from build123d import *

# Parameters (mm, degrees)
SKETCH1_R                                     = 50.8
BOSS_EXTRUDE1_DEPTH                           = 3.175
BOSS_EXTRUDE2_DEPTH                           = 3.175
FILLET1_R                                     = 3.175
CSK_FOR_8_FLAT_HEAD_SOCKET_CAP_SCREW1_A_COUNT = 2
CSK_FOR_8_FLAT_HEAD_SOCKET_CAP_SCREW1_A_PITCH = 23.8125
CSK_FOR_8_FLAT_HEAD_SOCKET_CAP_SCRE_2_COUNT   = 2
CSK_FOR_8_FLAT_HEAD_SOCKET_CAP_SCRE_2_PITCH   = 65.445830702
CSK_FOR_8_FLAT_HEAD_SOCKET_CAP_SCRE_3_COUNT   = 2
CSK_FOR_8_FLAT_HEAD_SOCKET_CAP_SCRE_3_PITCH   = 60.96
CIRPATTERN1_COUNT                             = 6
CSK_FOR_4_FLAT_HEAD_SOCKET_CAP_SCREW2_A_COUNT = 2
CSK_FOR_4_FLAT_HEAD_SOCKET_CAP_SCREW2_A_PITCH = 15.875
CSK_FOR_4_FLAT_HEAD_SOCKET_CAP_SCRE_2_COUNT   = 2
CSK_FOR_4_FLAT_HEAD_SOCKET_CAP_SCRE_2_PITCH   = 15.875
SKETCH17_W                                    = 12.7
SKETCH17_H                                    = 25.4
CUT_EXTRUDE2_DEPTH                            = 74.042253397
FILLET2_R                                     = 1.5875


with BuildPart() as part:
    # Sketch1 → Boss-Extrude1 (new body)
    with BuildSketch(Plane(origin=(0, 0, 0), x_dir=(1, 0, 0), z_dir=(0, 1, 0))):
        with Locations(Location((0, 0, 0), (0, 0, 270))):
            Circle(SKETCH1_R)
    extrude(amount=BOSS_EXTRUDE1_DEPTH)

    # Sketch8 → Boss-Extrude2 (add)
    with BuildSketch(Plane.XZ):
        with BuildLine():
            Line((-52.3875, -15.875), (-48.255822188, -15.875))
            ThreePointArc((-48.255822188, -15.875), (-50.8, 0), (-48.255822188, 15.875))
            Line((-48.255822188, 15.875), (-52.3875, 15.875))
            Line((-52.3875, 15.875), (-52.3875, -15.875))
        make_face()
    extrude(amount=-BOSS_EXTRUDE2_DEPTH)

    # Fillet1
    fillet1_edges = [part.edges().sort_by_distance(p)[0] for p in [
        (-48.255822188, 1.5875, 15.875),
        (-48.255822188, 1.5875, -15.875),
    ]]
    fillet(fillet1_edges, radius=FILLET1_R)

    # Sketch6 → CSK for #8 Flat Head Socket Cap Screw1 (revolve, cut)
    with BuildSketch(Plane(origin=(-44.45, 0, 11.90625), x_dir=(0, 0, -1), z_dir=(1, 0, 0))):
        Polygon((0, 0), (0, 3.175), (2.2479, 3.175), (2.2479, 2.658961536), (4.5593, 0), align=None)
    csk_for_8_flat_head_socket_cap_screw1 = revolve(axis=Axis((-44.45, -6.35, 11.90625), (0, 1, 0)), mode=Mode.SUBTRACT)

    # CSK for #8 Flat Head Socket Cap Screw1 a: CSK for #8 Flat Head Socket Cap Screw1 ×2
    with Locations(*[(0, 0, -i * CSK_FOR_8_FLAT_HEAD_SOCKET_CAP_SCREW1_A_PITCH) for i in range(1, CSK_FOR_8_FLAT_HEAD_SOCKET_CAP_SCREW1_A_COUNT)]):
        add(csk_for_8_flat_head_socket_cap_screw1, mode=Mode.SUBTRACT)

    # CSK for _8 Flat Head Socket Cap Scre 2: CSK for #8 Flat Head Socket Cap Screw1 ×2
    with Locations(*[Vector(0.9314573494796193, 0, -0.36385052714047633) * (i * CSK_FOR_8_FLAT_HEAD_SOCKET_CAP_SCRE_2_PITCH) for i in range(1, CSK_FOR_8_FLAT_HEAD_SOCKET_CAP_SCRE_2_COUNT)]):
        add(csk_for_8_flat_head_socket_cap_screw1, mode=Mode.SUBTRACT)

    # CSK for _8 Flat Head Socket Cap Scre 3: CSK for #8 Flat Head Socket Cap Screw1 ×2
    with Locations(*[(i * CSK_FOR_8_FLAT_HEAD_SOCKET_CAP_SCRE_3_PITCH, 0, 0) for i in range(1, CSK_FOR_8_FLAT_HEAD_SOCKET_CAP_SCRE_3_COUNT)]):
        add(csk_for_8_flat_head_socket_cap_screw1, mode=Mode.SUBTRACT)

    # Sketch10 → #8-32 Tapped Hole1 (revolve, cut)
    with BuildSketch(Plane(origin=(0, 3.175, -44.45), x_dir=(0, 0, 1), z_dir=(1, 0, 0))):
        Polygon((0, 0), (0, 11.705806461), (1.7272, 10.668), (1.7272, 0), align=None)
    f_8_32_tapped_hole1 = revolve(axis=Axis((0, 9.525, -44.45), (0, -1, 0)), mode=Mode.SUBTRACT)

    # CirPattern1: #8-32 Tapped Hole1 ×6 about axis
    cirpattern1_axis = Axis((0, 0, 0), (0, 1, 0))
    for i in range(1, CIRPATTERN1_COUNT):
        add(f_8_32_tapped_hole1.rotate(cirpattern1_axis, i * 360 / CIRPATTERN1_COUNT), mode=Mode.SUBTRACT)

    # Sketch15 → CSK for #4 Flat Head Socket Cap Screw2 (revolve, cut)
    with BuildSketch(Plane(origin=(-15.24, 3.175, 0), x_dir=(0, 0, 1), z_dir=(1, 0, 0))):
        Polygon((0, 0), (0, 3.175), (1.63195, 3.175), (1.63195, 1.848124365), (3.2385, 0), align=None)
    csk_for_4_flat_head_socket_cap_screw2 = revolve(axis=Axis((-15.24, 9.525, 0), (0, -1, 0)), mode=Mode.SUBTRACT)

    # CSK for #4 Flat Head Socket Cap Screw2 a: CSK for #4 Flat Head Socket Cap Screw2 ×2
    with Locations(*[(0, 0, -i * CSK_FOR_4_FLAT_HEAD_SOCKET_CAP_SCREW2_A_PITCH) for i in range(1, CSK_FOR_4_FLAT_HEAD_SOCKET_CAP_SCREW2_A_COUNT)]):
        add(csk_for_4_flat_head_socket_cap_screw2, mode=Mode.SUBTRACT)

    # CSK for _4 Flat Head Socket Cap Scre 2: CSK for #4 Flat Head Socket Cap Screw2 ×2
    with Locations(*[(0, 0, i * CSK_FOR_4_FLAT_HEAD_SOCKET_CAP_SCRE_2_PITCH) for i in range(1, CSK_FOR_4_FLAT_HEAD_SOCKET_CAP_SCRE_2_COUNT)]):
        add(csk_for_4_flat_head_socket_cap_screw2, mode=Mode.SUBTRACT)

    # Sketch17 → Cut-Extrude2 (cut, through all)
    with BuildSketch(Plane(origin=(0, 3.175, 0), x_dir=(1, 0, 0), z_dir=(0, 1, 0))):
        Rectangle(SKETCH17_W, SKETCH17_H)
    extrude(amount=-CUT_EXTRUDE2_DEPTH, mode=Mode.SUBTRACT)

    # Fillet2
    fillet2_edges = [part.edges().sort_by_distance(p)[0] for p in [
        (-6.35, 1.5875, 12.7),
        (-6.35, 1.5875, -12.7),
        (6.35, 1.5875, -12.7),
        (6.35, 1.5875, 12.7),
    ]]
    fillet(fillet2_edges, radius=FILLET2_R)


solid = part.part
The listing builds one solid part. Answer for the finished solid, in the listing's coordinates (mm). A direction names the side the tool comes from. Round coordinates to 2 decimals unless told otherwise and drop trailing zeros. Order: outer loops, then holes, each group sorted by start corner. A loop starts at its lowest first (then second) coordinate and runs counter-clockwise, first axis right, second up. Notation, with made-up numbers: (-2, 76.25) -> (33, 76.25) arc R27 cw to (33, 113.25) -> close; hole circle Ø10 at (31, 57.25). An arc over 180 degrees is marked (long way). Put each result on its own line as item: value.
Q1. Consider line 1 along X through (y, z) = (0.7, 0); line 2 along Z through (x, y) = (-15.24, 0.6); line 3 along X through (y, z) = (2.3, -44.45). Determine where each line is inside the solid, lowest interval first.
Results list:
line 1: -52.39 to -16.87, -13.61 to -6.35, 6.35 to 50.8
line 2: -48.46 to -17.51, -14.24 to -1.63, 1.63 to 14.24, 17.51 to 48.46
line 3: -24.59 to -1.73, 1.73 to 24.59
Q2. Section A-A, the plane x = 0 is taken. Write down the section's boundary in (y, z) (3 decimals), and give its area (3 significant figures).
Results list:
outline: (0, -50.8) -> (3.175, -50.8) -> (3.175, -46.177) -> (0, -46.177) -> close; (0, -42.723) -> (3.175, -42.723) -> (3.175, -12.7) -> (0, -12.7) -> close; (0, 12.7) -> (3.175, 12.7) -> (3.175, 42.723) -> (0, 42.723) -> close; (0, 46.177) -> (3.175, 46.177) -> (3.175, 50.8) -> (0, 50.8) -> close
area: 220 mm^2
Q3. Determine the mould class of faces 1 (the conical face through (-16.41, 1.44, 14.6)), 2 (the cylindrical face through (50.76, 1.57, 1.98)), 3 (the flat face through (11, 3.175, -1)) for opening direction Z: pulls with the +Z half, pulls with the -Z half, needs draft (parallel to the pull), parting line crosses it, or undercut.
Results list:
face 1: undercut
face 2: parting line crosses it
face 3: needs draft
Q4. Section C-C, the plane x = -44.45 is taken. Write down the section's boundary in (y, z) (3 decimals), and give its area (3 significant figures).
Results list:
outline: (0, -24.593) -> (3.175, -24.593) -> (3.175, -14.154) -> (2.659, -14.154) -> (0, -16.466) -> close; (0, -7.347) -> (2.659, -9.658) -> (3.175, -9.658) -> (3.175, 9.658) -> (2.659, 9.658) -> (0, 7.347) -> close; (0, 16.466) -> (2.659, 14.154) -> (3.175, 14.154) -> (3.175, 24.593) -> (0, 24.593) -> close
area: 115 mm^2
Q5. Section D-D, the plane z = 44.45 is taken. Write down the section's boundary in (x, y) (3 decimals).
Results list:
outline: (-24.593, 0) -> (-1.727, 0) -> (-1.727, 3.175) -> (-24.593, 3.175) -> close; (1.727, 0) -> (24.593, 0) -> (24.593, 3.175) -> (1.727, 3.175) -> close
Q6. Each of these flat-tipped pins is pushed along its axis until it touches: P1, Ø1, axis at x = 2, y = 1.5, coming from the +Z side; P2, Ø0.6, axis at x = -51.5, y = 1, coming from the +Z side (3 decimals); P3, Ø1.5, axis at y = 0.5, z = 33, coming from the -X side. Where does it stop, or does it pass through?
Results list:
P1: z = 50.78
P2: z = 15.875
P3: x = -39.25
Q7. Which of the six approach directions +Z, -Z, +X, -X, +Y, -Y give full straight-line access (tool end or side, diameter ignored) to faces 4 (the flat face through (0, 2, -12.7)), 5 (the conical face through (18.633, 2.493, -13.01))?
Results list:
face 4: +Y, -Y
face 5: -Y
Q8. Section B-B, the plane y = 1.9 is taken. Count the separate pieces of the cut face and the enclosed holes in it, and give its area (3 significant figures).
Results list:
separate pieces: 1
enclosed holes: 14
area: 7,660 mm^2
